For this review, take the finished solid that the model builds, in its own axes (mm). A direction names the side the tool comes from. Round coordinates to 2 decimals unless told otherwise and drop trailing zeros. Order: outer loops, then holes, each group sorted by start corner. A loop starts at its lowest first (then second) coordinate and runs counter-clockwise, first axis right, second up. Notation, with made-up numbers: (20.5, 11) - (62.5, 11) arc R25 ccw to (62.5, 33) - close; hole circle Ø10 at (86.25, 87). An arc over 180 degrees is marked (long way). One line per item, written item: value.
```python
from build123d import *

# Parameters (mm, degrees)
EXTRUDE_1_DEPTH     = 3
CUT_EXTRUDE_4_DEPTH = 4
SKETCH_12_R         = 15
SKETCH_12_R_2       = 6.125
EXTRUDE_2_DEPTH     = 2.6
SKETCH_13_R         = 15
SKETCH_13_R_2       = 7.25
EXTRUDE_3_DEPTH     = 1.1
SKETCH_14_R         = 1.2
CUT_EXTRUDE_5_DEPTH = 7.7
FILLET_1_R          = 1


with BuildPart() as part:
    # 스케치1 → 보스-돌출1 (new body)
    with BuildSketch(Plane.XY):
        with BuildLine():
            Line((-5, -6.9), (-6.9, -6.9))
            Line((-6.9, -6.9), (-6.9, 6.9))
            Line((-6.9, 6.9), (6.9, 6.9))
            Line((6.9, 6.9), (6.9, -6.9))
            Line((6.9, -6.9), (5, -6.9))
            Line((5, -6.9), (5, -14.142135624))
            ThreePointArc((5, -14.142135624), (0, 15), (-5, -14.142135624))
            Line((-5, -14.142135624), (-5, -6.9))
        make_face()
    extrude(amount=EXTRUDE_1_DEPTH)

    # 스케치11 → 컷-돌출4 (cut, through all)
    with BuildSketch(Plane.XY.offset(3)):
        with BuildLine():
            Line((5.8, -1.8), (-5.8, -1.8))
            ThreePointArc((-5.8, -1.8), (-7.6, 0), (-5.8, 1.8))
            Line((-5.8, 1.8), (5.8, 1.8))
            ThreePointArc((5.8, 1.8), (7.6, 0), (5.8, -1.8))
        make_face()
    extrude(amount=-CUT_EXTRUDE_4_DEPTH, mode=Mode.SUBTRACT)

    # 스케치12 → 보스-돌출2 (add)
    with BuildSketch(Plane.XY.offset(3)):
        Circle(SKETCH_12_R)
        Circle(SKETCH_12_R_2, mode=Mode.SUBTRACT)
    extrude(amount=EXTRUDE_2_DEPTH)

    # 스케치13 → 보스-돌출3 (add)
    with BuildSketch(Plane.XY.offset(5.6)):
        Circle(SKETCH_13_R)
        Circle(SKETCH_13_R_2, mode=Mode.SUBTRACT)
    extrude(amount=EXTRUDE_3_DEPTH)

    # 스케치14 → 컷-돌출5 (cut, through all)
    with BuildSketch(Plane.XY.offset(6.7)):
        with Locations((10.825317547, 6.25)):
            Circle(SKETCH_14_R)
        with Locations((-10.825317547, 6.25)):
            Circle(SKETCH_14_R)
        with Locations((10.825317547, -6.25)):
            Circle(SKETCH_14_R)
        with Locations((-10.825317547, -6.25)):
            Circle(SKETCH_14_R)
    extrude(amount=-CUT_EXTRUDE_5_DEPTH, mode=Mode.SUBTRACT)

    # 필렛1
    fillet_1_edges = [part.edges().sort_by_distance(p)[0] for p in [
        (-5, -6.9, 1.5),
        (5, -6.9, 1.5),
    ]]
    fillet(fillet_1_edges, radius=FILLET_1_R)


solid = part.part
```
Item 1: Take a section at B-B (x = 0). Write out the cut boundary in (y, z) (3 decimals).
Returned:
outline: (-15, 3) - (-6.125, 3) - (-6.125, 5.6) - (-7.25, 5.6) - (-7.25, 6.7) - (-15, 6.7) - close; (6.125, 3) - (6.9, 3) - (6.9, 0) - (15, 0) - (15, 6.7) - (7.25, 6.7) - (7.25, 5.6) - (6.125, 5.6) - close
Item 2: For P1, Ø0.9, axis at y = -4, z = 1, coming from the +X side; P2, Ø1, axis at x = 6.5, z = 1.5, coming from the +Y side; P3, Ø0.9, axis at x = -2, z = 2, coming from the -Y side, all flat-tipped, find the tip position at first contact; note any pin that passes through.
Returned:
P1: x = 14.57
P2: y = 13.75
P3: y = 6.9
Item 3: Wall thickness on line 1 (Y direction, x = 11, z = 3.25); line 2 (Y direction, x = 0, z = 3.5) (3 decimals); line 3 (Y direction, x = -10, z = 1.25): over which ranges is each line inside the solid? List them lowest first.
Returned:
line 1: -10.2 to -7.44, -5.06 to 5.06, 7.44 to 10.2
line 2: -15 to -6.125, 6.125 to 15
line 3: -11.18 to -7.12, -5.38 to 5.38, 7.12 to 11.18
Item 4: The part is to be moulded in two halves that separate along X. For faces 1 (the cylindrical face through (13.373, -6.794, 2.559)), 2 (the flat face through (-0.2, 7.1, 0)), 3 (the cylindrical face through (12, -6, 3)), say which applies: +X half, -X half, draft (parallel to the pull), parting line (faces both ways), or undercut.
Returned:
face 1: parting line
face 2: draft
face 3: undercut
Item 5: Take a section at A-A (z = 1.25). Write out the cut boundary in (x, y), plus the area to 3 significant figures.
Returned:
outline: (-6.9, -6.9) - (-6.9, -1.42) arc R1.8 cw to (-6.9, 1.42) - (-6.9, 6.9) - (6.9, 6.9) - (6.9, 1.42) arc R1.8 cw to (6.9, -1.42) - (6.9, -6.9) - (6, -6.9) arc R1 ccw to (5, -7.9) - (5, -14.14) arc R15 ccw (long way) to (-5, -14.14) - (-5, -7.9) arc R1 ccw to (-6, -6.9) - close; hole circle Ø2.4 at (-10.83, -6.25); hole circle Ø2.4 at (-10.83, 6.25); hole circle Ø2.4 at (10.83, -6.25); hole circle Ø2.4 at (10.83, 6.25)
area: 417 mm^2
Item 6: Take a section at D-D (z = 4). Write out the cut boundary in (x, y) (3 decimals).
Returned:
outline: circle Ø30 at (0, 0); hole circle Ø2.4 at (-10.825, -6.25); hole circle Ø2.4 at (-10.825, 6.25); hole circle Ø12.25 at (0, 0); hole circle Ø2.4 at (10.825, -6.25); hole circle Ø2.4 at (10.825, 6.25)
Item 7: Machinability: for faces 4 (the flat face through (-2, 6, 5.6)), 5 (the flat face through (-5, -11, 1)), 6 (the cylindrical face through (7.6, 0, 1.5)), which of the approach directions +Z, -Z, +X, -X, +Y, -Y give a long, thin tool a straight path to every point of the face, cutting with its end or side? Answer none if there is none.
Returned:
face 4: +Z
face 5: -Z, -Y
face 6: -Z
